Could you check a few things on this drawing? It's one solid part, dimensions in mm from its lowest x, y, z. A direction names the side the tool comes from. Give positions to 0.01 mm unless a question says otherwise; leave off trailing zeros. Loops run counter-clockwise (first coordinate to the right, second up) from the corner with the lowest first, then second, coordinate; pieces in that order, holes last. Notation, with made-up numbers: (-28, -26) -> (-13, -26) arc R21 ccw to (-13, -8) -> close; hole circle Ø3 at (85, 86). An arc over 180 degrees is marked (long way). Use CSV: the item, a comma, the result in double quotes.
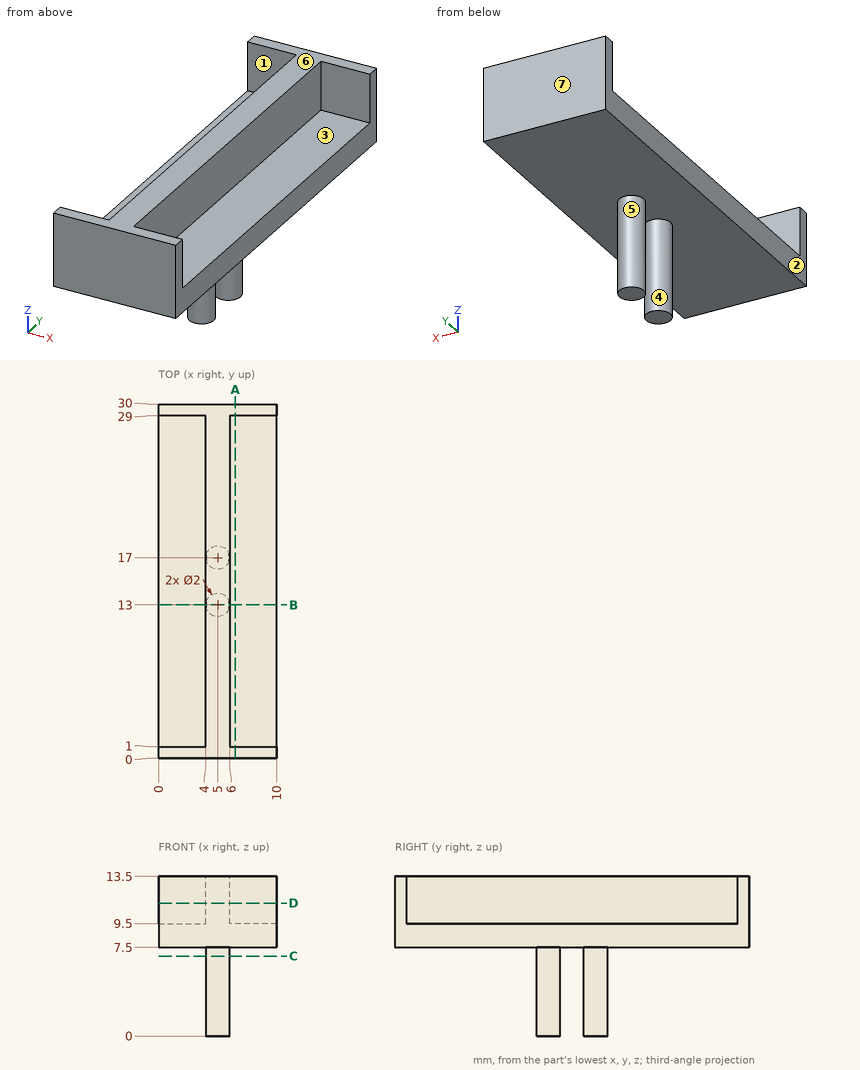
(1) If we section it at D-D, the plane z = 11.25: Write out the boundary of the cut face in (x, y).
Answer sheet:
outline,"(0, 0) -> (10, 0) -> (10, 1) -> (6, 1) -> (6, 29) -> (10, 29) -> (10, 30) -> (0, 30) -> (0, 29) -> (4, 29) -> (4, 1) -> (0, 1) -> close"
(2) If we section it at A-A, the plane x = 6.5: Write out the boundary of the cut face in (y, z), then the cut area to 3 significant figures.
Answer sheet:
outline,"(0, 7.5) -> (30, 7.5) -> (30, 13.5) -> (29, 13.5) -> (29, 9.5) -> (1, 9.5) -> (1, 13.5) -> (0, 13.5) -> close"
area,"68.0 mm2"
(3) If we section it at B-B, the plane y = 13: Write out the boundary of the cut face in (x, z).
Answer sheet:
outline,"(0, 7.5) -> (4, 7.5) -> (4, 0) -> (6, 0) -> (6, 7.5) -> (10, 7.5) -> (10, 9.5) -> (6, 9.5) -> (6, 13.5) -> (4, 13.5) -> (4, 9.5) -> (0, 9.5) -> close"
(4) Which directions (+Z, -Z, +X, -X, +Y, -Y) give clear straight access to the entire face, cutting with the end or side of a thin tool? Please do the marked faces 1, 2, 3 and 4.
Answer sheet:
face 1,"+Z, -X"
face 2,"+Z, -Z, -X, +Y, -Y"
face 3,"+Z, +X"
face 4,"-Z"
(5) We'd pull the mould along Y, two halves only. Please class the marked faces 5, 6 and 7: released by +Y, released by -Y, zero draft, split by the parting line, or undercut.
Answer sheet:
face 5,"undercut"
face 6,"zero draft"
face 7,"released by +Y"
(6) If I drill on L1, parallel to Y at x = 5, z = 1; L2, parallel to Y at x = 3.75, z = 11.25; L3, parallel to Z at x = 5, y = 1.75, over which ranges is the centre line in solid material (lowest first)? Write a range as from..to.
Answer sheet:
L1,"y = 12..14, 16..18"
L2,"y = 0..1, 29..30"
L3,"z = 7.5..13.5"
(7) Will these pins go through, and if not, where does the flat tip stop? pin 1 Ø4.5 at (x, y) = (7, 9) entering from +Z; pin 2 Ø1.5 at (y, z) = (26, 11.5) entering from -X; pin 3 Ø4 at (x, y) = (1, 11) entering from +Z; pin 4 Ø3 at (x, y) = (7.5, 11.5) entering from -Z.
Answer sheet:
pin 1,"stops at z = 13.5"
pin 2,"stops at x = 4"
pin 3,"stops at z = 9.5"
pin 4,"stops at z = 7.5"
(8) If we section it at C-C, the plane z = 6.75: Write out the boundary of the cut face in (x, y), then the cut area to 3 significant figures.
Answer sheet:
outline,"circle Ø2 at (5, 13); circle Ø2 at (5, 17)"
area,"6.28 mm2"
